Design review of the part built by this model. Coordinates are the model's own, in mm. A direction names the side the tool comes from. Coordinates: 2 decimals unless noted, no trailing zeros. Loops run counter-clockwise (first coordinate to the right, second up) from the corner with the lowest first, then second, coordinate; pieces in that order, holes last. Notation, with made-up numbers: M 40,-34.5 L 65,-34.5 A14 ccw 65,-30.5 Z; hole C 88.25,67.25 d7. An arc over 180 degrees is marked long. Write item = value, one per line. Start each with the question number.
from build123d import *

# Parameters (mm, degrees)
SKETCH1_R                     = 43.815
HOUSING_FITTING_EXTRUDE_DEPTH = 17.018
HOUSING_BODY_1_DEPTH          = 19.05
SKETCH3_R                     = 6.35
IMPELLER_BORE_DEPTH           = 17.018
SKETCH4_R                     = 4
SHAFT_BORE_DEPTH              = 70.612
O_RING_CUT_DEPTH              = 1.27
O_RING_CUT_DEPTH_BACK         = 1.27
SKETCH5_R                     = 43.942
SKETCH5_R_2                   = 43.18
SKETCH12_R                    = 3.175
CUT_EXTRUDE2_DEPTH            = 19.05
CIRPATTERN1_COUNT             = 8
SKETCH14_R                    = 3.175
SKETCH14_R_2                  = 3.392842108
CUT_EXTRUDE4_DEPTH            = 16.51
SKETCH15_R                    = 3.175
CUT_EXTRUDE5_DEPTH            = 10.922
FILLET1_R                     = 6.604
SKETCH16_R                    = 12.954
CUT_EXTRUDE7_DEPTH            = 28.448
SKETCH17_R                    = 15.24
CUT_EXTRUDE8_DEPTH            = 13.97
SKETCH20_R                    = 25.146
CUT_EXTRUDE11_DEPTH           = 6.35


with BuildPart() as part:
    # Sketch1 → Housing Fitting Extrude (new body)
    with BuildSketch(Plane(origin=(0, 0, 0), x_dir=(0, 0, -1), z_dir=(1, 0, 0))):
        Circle(SKETCH1_R)
    extrude(amount=HOUSING_FITTING_EXTRUDE_DEPTH)

    # Sketch2 → Housing Body 1 (add)
    with BuildSketch(Plane.ZY):
        with BuildLine():
            Line((60.96, 0), (60.96, 60.96))
            Line((60.96, 60.96), (0, 60.96))
            ThreePointArc((0, 60.96), (-43.105229381, 43.105229381), (-60.96, 0))
            Line((-60.96, 0), (-60.96, -54.61))
            Line((-60.96, -54.61), (-60.96, -60.96))
            Line((-60.96, -60.96), (60.96, -60.96))
            Line((60.96, -60.96), (60.96, -54.61))
            Line((60.96, -54.61), (60.96, 0))
        make_face()
    extrude(amount=HOUSING_BODY_1_DEPTH)

    # Sketch3 → Impeller Bore (cut)
    with BuildSketch(Plane(origin=(17.018, 0, 0), x_dir=(0, 0, -1), z_dir=(1, 0, 0))):
        Circle(SKETCH3_R)
    extrude(amount=-IMPELLER_BORE_DEPTH, mode=Mode.SUBTRACT)

    # Sketch4 → Shaft Bore (cut)
    with BuildSketch(Plane(origin=(0, 0, 0), x_dir=(0, 0, -1), z_dir=(1, 0, 0))):
        Circle(SKETCH4_R)
    extrude(amount=-SHAFT_BORE_DEPTH, mode=Mode.SUBTRACT)

    # Sketch5 → O-Ring Cut (cut, two sides: drawn at the far end of the back side and taken through both)
    with BuildSketch(Plane(origin=(8.509, 0, 0), x_dir=(0, 0, -1), z_dir=(1, 0, 0)).offset(-O_RING_CUT_DEPTH_BACK)):
        Circle(SKETCH5_R)
        Circle(SKETCH5_R_2, mode=Mode.SUBTRACT)
    extrude(amount=O_RING_CUT_DEPTH + O_RING_CUT_DEPTH_BACK, mode=Mode.SUBTRACT)

    # Sketch12 → Cut-Extrude2 (cut)
    with BuildSketch(Plane(origin=(0, 0, 0), x_dir=(0, 0, -1), z_dir=(1, 0, 0))):
        with Locations((-50.419, 0)):
            Circle(SKETCH12_R)
    cut_extrude2 = extrude(amount=-CUT_EXTRUDE2_DEPTH, mode=Mode.SUBTRACT)

    # CirPattern1: Cut-Extrude2 ×8 about axis, 1 skipped
    cirpattern1_axis = Axis((0, 0, 0), (1, 0, 0))
    add([cut_extrude2.rotate(cirpattern1_axis, i * 360 / CIRPATTERN1_COUNT) for i in range(1, CIRPATTERN1_COUNT) if i not in (7,)], mode=Mode.SUBTRACT)

    # Sketch14 → Cut-Extrude4 (cut)
    with BuildSketch(Plane.XZ.offset(60.96)):
        with Locations(Location((-9.525, -46.754349092, 0), (0, 0, 270))):
            Circle(SKETCH14_R)
        with Locations(Location((-9.525, 41.914080666, 0), (0, 0, 270))):
            Circle(SKETCH14_R_2)
    extrude(amount=-CUT_EXTRUDE4_DEPTH, mode=Mode.SUBTRACT)

    # Sketch15 → Cut-Extrude5 (cut)
    with BuildSketch(Plane(origin=(0, 0, -60.96), x_dir=(-1, 0, 0), z_dir=(0, 0, -1))):
        with Locations(Location((9.525, -39.337514031, 0), (0, 0, 90))):
            Circle(SKETCH15_R)
    extrude(amount=-CUT_EXTRUDE5_DEPTH, mode=Mode.SUBTRACT)

    # Fillet1
    fillet1_edges = [part.edges().sort_by_distance(p)[0] for p in [
        (17.018, 0, 6.35),
    ]]
    fillet(fillet1_edges, radius=FILLET1_R)

    # Sketch16 → Cut-Extrude7 (cut)
    with BuildSketch(Plane.ZY.offset(19.05)):
        Circle(SKETCH16_R)
    extrude(amount=-CUT_EXTRUDE7_DEPTH, mode=Mode.SUBTRACT)

    # Sketch17 → Cut-Extrude8 (cut)
    with BuildSketch(Plane.ZY.offset(19.05)):
        Circle(SKETCH17_R)
    extrude(amount=-CUT_EXTRUDE8_DEPTH, mode=Mode.SUBTRACT)

    # Sketch20 → Cut-Extrude11 (cut)
    with BuildSketch(Plane.ZY.offset(19.05)):
        Circle(SKETCH20_R)
    extrude(amount=-CUT_EXTRUDE11_DEPTH, mode=Mode.SUBTRACT)


solid = part.part
Q1. Add section A-A on z = 36. State the section outline as (x, y) points, plus the area to 3 significant figures.
Q2. Add section C-C on z = -22. State the section outline as (x, y) points.
Q3. To check wall thickness, follow line 1 (Z direction, x = -10, y = -45.5); line 2 (Y direction, x = 1.75, z = 0) (3 decimals); line 3 (X direction, y = 50, z = 41.5). State the ranges of each line that lie inside material, in increasing order. Write a range as from..to.
Q4. Clearance check with flat-ended pins moving along their axes: P1, Ø12, axis at y = 35, z = -40.5, coming from the +X side; P2, Ø6, axis at x = 5.5, z = 6, coming from the -Y side; P3, Ø25, axis at y = -3.5, z = 3, coming from the -X side. State where each tip first meets the part, or that it passes through.
Q5. Mouldability with a two-part tool opening along Z and no side actions: class faces 1 (the face through (-12.7, -11, 11)), 2 (the face through (0, -40, 26)), 3 (the face through (-8.506, -52.821, 38.678)), 4 (the face through (-9, -39, -50.038)) as released by +Z, released by -Z, zero draft, split by the parting line, or undercut.
Q6. Add section B-B on y = -20. State the section outline as (x, z) points, plus the area to 3 significant figures.
Q7. For faces 5 (the face through (9.779, -29, -32.3)), 6 (the face through (9.91, -6.2, 1.38)), 7 (the face through (-5.08, -11.22, -6.84)), list the 3-axis set-ups (+Z, -Z, +X, -X, +Y, -Y) from which the entire face can be reached by the end or side of a thin tool; tool diameter is ignored.
Values follow:
q1.outline = M -19.05,-60.96 L 0,-60.96 L 0,-38.81 L -19.05,-38.81 Z; M -19.05,-32.5 L 0,-32.5 L 0,-24.98 L 7.24,-24.98 L 7.24,-23.84 L 9.78,-23.84 L 9.78,-24.98 L 17.02,-24.98 L 17.02,24.98 L 9.78,24.98 L 9.78,23.84 L 7.24,23.84 L 7.24,24.98 L 0,24.98 L 0,60.96 L -19.05,60.96 Z
q1.area = 3,050 mm2
q2.outline = M -19.05,-60.96 L 0,-60.96 L 0,-37.89 L 7.24,-37.89 L 7.24,-37.16 L 9.78,-37.16 L 9.78,-37.89 L 17.02,-37.89 L 17.02,37.89 L 9.78,37.89 L 9.78,37.16 L 7.24,37.16 L 7.24,37.89 L 0,37.89 L 0,56.85 L -19.05,56.85 L -19.05,12.18 L -12.7,12.18 L -12.7,-12.18 L -19.05,-12.18 Z
q3.line_1 = -60.96..-49.89, -43.62..38.55, 45.27..60.96
q3.line_2 = -43.815..-12.954, 12.954..43.815
q3.line_3 = -19.05..0
q4.P1 = 0
q4.P2 = -43.71
q4.P3 = -12.7
q5.face_1 = undercut
q5.face_2 = zero draft
q5.face_3 = undercut
q5.face_4 = released by -Z
q6.outline = M -19.05,-60.96 L 0,-60.96 L 0,-38.98 L 7.24,-38.98 L 7.24,-38.27 L 9.78,-38.27 L 9.78,-38.98 L 17.02,-38.98 L 17.02,38.98 L 9.78,38.98 L 9.78,38.27 L 7.24,38.27 L 7.24,38.98 L 0,38.98 L 0,60.96 L -19.05,60.96 L -19.05,15.24 L -12.7,15.24 L -12.7,-15.24 L -19.05,-15.24 Z
q6.area = 3,450 mm2
q7.face_5 = none
q7.face_6 = +X, -X
q7.face_7 = -X
